Design review of the part built by this model. Coordinates are the model's own, in mm. Face numbers are marked on the shaded views. A direction names the side the tool comes from. Round coordinates to 2 decimals unless told otherwise and drop trailing zeros. Write each loop counter-clockwise with the first axis right and the second up, starting at its lowest first coordinate (ties: lowest second). Pieces come first, ordered by that corner, then holes. Notation, with made-up numbers: (60, 75) -> (79, 75) arc R15 ccw to (79, 96) -> close; hole circle Ø11 at (64, -11). An arc over 180 degrees is marked (long way). Write item = value, one per line. Start each with the question number.
Item 1: Add section D-D, the plane x = 11. State the section outline as (y, z) points.
Item 2: Add section A-A, the plane y = -20. State the section outline as (x, z) points (3 decimals), then the cut area to 3 significant figures.
Item 3: Add section B-B, the plane x = 6. State the section outline as (y, z) points, then the cut area to 3 significant figures.
Item 4: Machinability: for the marked faces 1, 2 and 3, which of the approach directions +Z, -Z, +X, -X, +Y, -Y give a long, thin tool a straight path to every point of the face, cutting with its end or side? Answer none if there is none.
Item 5: For pin 1 Ø1.9 at (x, z) = (21.5, 4.5) entering from -Y; pin 2 Ø7 at (y, z) = (-18.5, 3) entering from +X; pin 3 Ø6 at (x, z) = (8, 5.5) entering from -Y; pin 4 Ø1 at (y, z) = (-10, 3.5) entering from +X, all flat-tipped, find the tip position at first contact; note any pin that passes through.
Item 6: To check wall thickness, follow L1, parallel to Z at x = 14.75, y = -34; L2, parallel to X at y = -23.5, z = 0.5; L3, parallel to Y at x = 4.25, z = 15.5. State the ranges of each line that lie inside material, in increasing order.
Item 7: Add section C-C, the plane z = 8.25. State the section outline as (x, y) points, then the cut area to 3 significant figures.
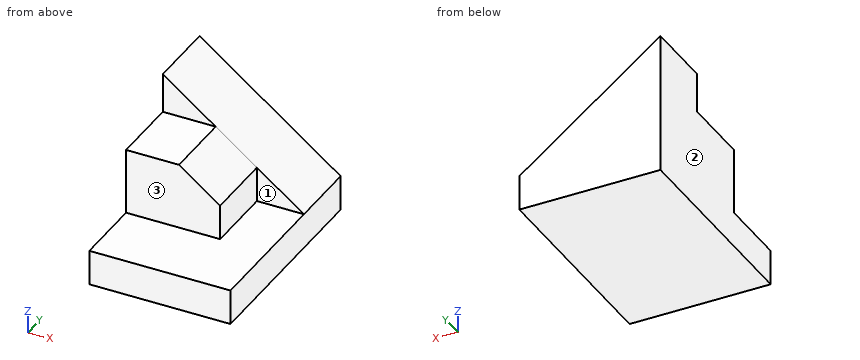
from build123d import *

# Parameters (mm, degrees)
F0_W     = 25.4
F0_H     = 6.35
F1_DEPTH = 38.1
F2_DEPTH = 12.7
F4_DEPTH = 12.7


with BuildPart() as f1:
    # F0 (on Front) → F1 (new body)
    with BuildSketch(Plane.XZ):
        with Locations((12.7, -3.175)):
            Rectangle(F0_W, F0_H)
    extrude(amount=F1_DEPTH)

    # F0 (on Front) → F2 (join)
    with BuildSketch(Plane.XZ):
        Polygon((0, 19.05), (0, 0), (25.4, 0), align=None)
    extrude(amount=F2_DEPTH)

    # F3 (on face) → F4 (join)
    with BuildSketch(Plane.XZ.offset(12.7)):
        Polygon((0, 11.90625), (0, 0), (16.933333, 0), (16.933333, 6.35), (9.525, 11.90625), align=None)
    extrude(amount=F4_DEPTH)


solid = f1.part
Result set:
q1.outline = (-38.1, -6.35) -> (0, -6.35) -> (0, 10.8) -> (-25.4, 10.8) -> (-25.4, 0) -> (-38.1, 0) -> close
q2.outline = (0, -6.35) -> (25.4, -6.35) -> (25.4, 0) -> (16.933, 0) -> (16.933, 6.35) -> (9.525, 11.906) -> (0, 11.906) -> close
q2.area = 342 mm²
q3.outline = (-38.1, -6.35) -> (0, -6.35) -> (0, 14.55) -> (-12.7, 14.55) -> (-12.7, 11.91) -> (-25.4, 11.91) -> (-25.4, 0) -> (-38.1, 0) -> close
q3.area = 578 mm²
q4.face_1 = +Z, +X, -Y
q4.face_2 = +Z, -Z, -X, +Y, -Y
q4.face_3 = +Z, +X, -X, -Y
q5.pin_1 = through
q5.pin_2 = 25.4
q5.pin_3 = -25.4
q5.pin_4 = 21.4
q6.L1 = -6.35 to 0
q6.L2 = 0 to 16.93
q6.L3 = -12.7 to 0
q7.outline = (0, -25.4) -> (14.4, -25.4) -> (14.4, 0) -> (0, 0) -> close
q7.area = 366 mm²
